from build123d import *

# Parameters (mm, degrees)
SKETCH1_R           = 10.16
BOSS_EXTRUDE1_DEPTH = 127
BOSS_EXTRUDE2_DEPTH = 12.7
BOSS_EXTRUDE3_DEPTH = 12.7


with BuildPart() as part:
    # Sketch1 → Boss-Extrude1 (new body)
    with BuildSketch(Plane(origin=(0, 0, 0), x_dir=(1, 0, 0), z_dir=(0, 1, 0))):
        Circle(SKETCH1_R)
    extrude(amount=BOSS_EXTRUDE1_DEPTH)

    # Sketch2 → Boss-Extrude2 (add)
    with BuildSketch(Plane(origin=(0, 127, 0), x_dir=(1, 0, 0), z_dir=(0, 1, 0))):
        Polygon((0, 15.24), (-13.198227154, 7.62), (-13.198227154, -7.62), (0, -15.24), (13.198227154, -7.62), (13.198227154, 7.62), align=None)
    extrude(amount=BOSS_EXTRUDE2_DEPTH)

    # Sketch3 → Boss-Extrude3 (add)
    with BuildSketch(Plane.XZ):
        Polygon((-13.198227154, 7.62), (-13.198227154, -7.62), (0, -15.24), (13.198227154, -7.62), (13.198227154, 7.62), (0, 15.24), align=None)
    extrude(amount=BOSS_EXTRUDE3_DEPTH)


solid = part.part
Geometry: final body of the model. Coordinates: model frame, mm. A direction names the side the tool comes from. Give positions to 0.01 mm unless a question says otherwise; leave off trailing zeros. Loops run counter-clockwise (first coordinate to the right, second up) from the corner with the lowest first, then second, coordinate; pieces in that order, holes last. Notation, with made-up numbers: (20, 36.5) - (65, 36.5) arc R15 cw to (65, 63.5) - close; hole circle Ø4 at (33, -32.75). An arc over 180 degrees is marked (long way). Answer as CSV lines item,"result". Start each with the question number.
1. Pin query (flat end, axial travel): P1, Ø2, axis at x = 1.5, y = 4, coming from the +Z side; P2, Ø5, axis at x = -3.5, y = 60, coming from the -Z side; P3, Ø1, axis at x = -9.5, y = 98, coming from the +Z side. Return the tip coordinate at first contact, or that it passes through.
2. Section C-C, the plane y = 110. Return loops of the section in (x, z).
3. Section B-B, the plane x = 7. Return loops of the section in (y, z).
4. Section A-A, the plane z = 4. Return loops of the section in (x, y).
5. Reachability of faces 1 (the face through (13.198, 133, 0)), 2 (the face through (-1.323, 62.611, -10.074)) from +Z, -Z, +X, -X, +Y, -Y: full face, straight path, thin tool, end or side. Return the list, or none.
6. Ray query, L1, parallel to Y at x = -3.5, z = 12; L2, parallel to Z at x = 0.25, y = 60; L3, parallel to X at y = 4, z = -7. Return the intervals inside material, ascending.
7. Draft query along Y for faces 3 (the face through (0, 139.7, 0)), 4 (the face through (-4.9, 0, 9.1)), 5 (the face through (-4.9, 127, -9.1)), 6 (the face through (-13.198, -6, 0)). Return one class per face: released by +Y, released by -Y, zero draft, split by the parting line, or undercut.
Answers:
1,P1,"stops at z = 10.15"
1,P2,"stops at z = -10.11"
1,P3,"stops at z = 4.71"
2,outline,"circle Ø20.32 at (0, 0)"
3,outline,"(-12.7, -11.2) - (0, -11.2) - (0, -7.36) - (127, -7.36) - (127, -11.2) - (139.7, -11.2) - (139.7, 11.2) - (127, 11.2) - (127, 7.36) - (0, 7.36) - (0, 11.2) - (-12.7, 11.2) - close"
4,outline,"(-13.2, -12.7) - (13.2, -12.7) - (13.2, 0) - (9.34, 0) - (9.34, 127) - (13.2, 127) - (13.2, 139.7) - (-13.2, 139.7) - (-13.2, 127) - (-9.34, 127) - (-9.34, 0) - (-13.2, 0) - close"
5,face 1,"+Z, -Z, +X, +Y, -Y"
5,face 2,"none"
6,L1,"y = -12.7 to 0, 127 to 139.7"
6,L2,"z = -10.16 to 10.16"
6,L3,"x = -7.36 to 7.36"
7,face 3,"released by +Y"
7,face 4,"undercut"
7,face 5,"undercut"
7,face 6,"zero draft"
